Build history of the part. All positions in model axes, mm. Face numbers are marked on the shaded views. A direction names the side the tool comes from. Round coordinates to 2 decimals unless told otherwise and drop trailing zeros. Write each loop counter-clockwise with the first axis right and the second up, starting at its lowest first coordinate (ties: lowest second). Pieces come first, ordered by that corner, then holes. Notation, with made-up numbers: M 51.25,75.5 L 107.25,75.5 A16 cw 107.25,96.5 Z; hole C 86.25,58.25 d8. An arc over 180 degrees is marked long. Use a Markdown table: item, result.
from build123d import *

# Parameters (mm, degrees)
BOSS_EXTRUDE2_DEPTH = 6.35
SHELL3_T            = -1.27
SKETCH2_7_R         = 4.7625
SKETCH2_7_R_2       = 3.175
CUT_EXTRUDE2_DEPTH  = 30.315069184
BOSS_EXTRUDE3_DEPTH = 0.635
DRAFT2_ANGLE        = 10


with BuildPart() as part:
    # Sketch2 → Boss-Extrude2 (new body)
    with BuildSketch(Plane(origin=(0, 0, 0), x_dir=(0, 1, 0), z_dir=(0, 0, 1))):
        with BuildLine():
            Line((8.659090909, -13.305478933), (20.926136364, -5.322191573))
            ThreePointArc((20.926136364, -5.322191573), (23.8125, 0), (20.926136364, 5.322191573))
            Line((20.926136364, 5.322191573), (8.659090909, 13.305478933))
            ThreePointArc((8.659090909, 13.305478933), (-15.875, 0), (8.659090909, -13.305478933))
        make_face()
    extrude(amount=BOSS_EXTRUDE2_DEPTH)

    # Shell3
    shell3_openings = [part.faces().sort_by_distance(p)[0] for p in [
        (0, 2.303090429, 6.35),
    ]]
    offset(amount=SHELL3_T, openings=shell3_openings, kind=Kind.INTERSECTION)

    # Sketch2<7> → Cut-Extrude2 (cut, through all)
    with BuildSketch(Plane(origin=(0, 0, 0), x_dir=(0, 1, 0), z_dir=(0, 0, 1))):
        with Locations(Location((0, 0, 0), (0, 0, 270))):
            Circle(SKETCH2_7_R)
        with Locations(Location((17.4625, 0, 0), (0, 0, 270))):
            Circle(SKETCH2_7_R_2)
    extrude(amount=CUT_EXTRUDE2_DEPTH, mode=Mode.SUBTRACT)

    # Sketch6 → Boss-Extrude3 (add)
    with BuildSketch(Plane(origin=(0, 0, 5.715), x_dir=(0, -1, 0), z_dir=(0, 0, 1))):
        Polygon((-16.769772727, 8.027117173), (-17.4625, 9.091555487), (-14.269185056, 11.169737305), (-13.576457783, 10.105298991), align=None)
        Polygon((-14.269185056, -11.169737305), (-13.576457783, -10.105298991), (-16.769772727, -8.027117173), (-17.4625, -9.091555487), align=None)
    extrude(amount=BOSS_EXTRUDE3_DEPTH)

    # Draft2
    draft2_faces = [part.faces().sort_by_distance(p)[0] for p in [
        (10.130646396, 15.865842528, 6.0325),
        (-10.130646396, 15.865842528, 6.0325),
    ]]
    draft(draft2_faces, Plane(origin=(0, 17.4625, 6.35), x_dir=(1, 0, 0), z_dir=(0, 0, 1)), DRAFT2_ANGLE)


solid = part.part
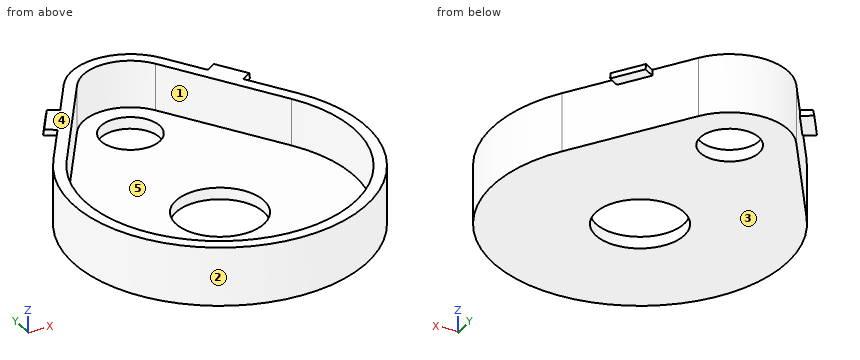
Q1. Which spindle directions (+Z, -Z, +X, -X, +Y, -Y) get a long thin tool onto all of the face, cutting with end or side? Do the marked faces 4 and 5. Say none if no direction does.
Response values:
| item | result |
|---|---|
| face 4 | +Z, +X, -X, +Y, -Y |
| face 5 | +Z |
Q2. Drill centre lines: L1, parallel to Y at x = 0, z = 0.85 (1 decimal); L2, parallel to X at y = 0, z = 5.1 (3 decimals); L3, parallel to Y at x = -1, z = 0.5. Where is each one in solid material? Low to high.
Response values:
| item | result |
|---|---|
| L1 | y = -15.9 to -4.8, 4.8 to 14.3, 20.6 to 23.8 |
| L2 | x = -15.875 to -14.605, 14.605 to 15.875 |
| L3 | y = -15.84 to -4.66, 4.66 to 14.45, 20.48 to 23.73 |
Q3. Cut at C-C on y = -6. Give the cut face in (x, z).
Response values:
| item | result |
|---|---|
| outline | M -14.7,0 L 14.7,0 L 14.7,6.35 L 13.32,6.35 L 13.32,1.27 L -13.32,1.27 L -13.32,6.35 L -14.7,6.35 Z |
Q4. Two-plate mould, pull along X, no slides. Class the marked faces 1, 2 and 3: +X half, -X half, draft (parallel to the pull), parting line (faces both ways), or undercut.
Response values:
| item | result |
|---|---|
| face 1 | undercut |
| face 2 | parting line |
| face 3 | draft |
Q5. Cut at B-B on x = 0. Count the separate pieces of the cut face and the enclosed holes in it, and give its area (3 significant figures).
Response values:
| item | result |
|---|---|
| separate pieces | 3 |
| enclosed holes | 0 |
| area | 43.1 mm2 |
Q6. Drop flat-ended pins along their axis: P1, Ø2, axis at x = 2.5, y = 19, coming from the +Z side; P2, Ø1.5, axis at y = 9, z = 2, coming from the +X side; P3, Ø5, axis at x = 0, y = 17.46, coming from the -Z side; P4, Ø3, axis at y = 14, z = 3, coming from the -X side. Give the stop position or say it passes through.
Response values:
| item | result |
|---|---|
| P1 | stops at z = 1.27 |
| P2 | stops at x = 13.56 |
| P3 | passes through |
| P4 | stops at x = -10.81 |
